```python
from build123d import *

# Parameters (mm, degrees)
SZKIC1_R                          = 10
DODANIE_WYCI_GNI_CIE1_DEPTH       = 357.5
SZKIC2_R                          = 8
DODANIE_WYCI_GNI_CIE2_DEPTH       = 32
SFAZOWANIE1_SIZE                  = 1.5
SFAZOWANIE2_SIZE2                 = 1.154700538
SFAZOWANIE2_SIZE                  = 2
SZKIC3_W                          = 28.491583868
SZKIC3_H                          = 26.39290166
SZKIC3_W_2                        = 17
SZKIC3_H_2                        = 17
WYTNIJ_WYCI_GNI_CIE1_DEPTH        = 5
SFAZOWANIE3_SIZE                  = 1
OTW_R_GWINTOWANY_M121_D           = 10.2
OTW_R_GWINTOWANY_M121_DEPTH       = 18
OTW_R_GWINTOWANY_M121_CSINK_D     = 13
OTW_R_GWINTOWANY_M121_CSINK_ANGLE = 90
OTW_R_GWINTOWANY_M121_TIP         = 3.064389157


with BuildPart() as part:
    # Szkic1 → Dodanie-wyciągnięcie1 (new body)
    with BuildSketch(Plane(origin=(0, 0, 0), x_dir=(0, 0, -1), z_dir=(1, 0, 0))):
        with Locations((-94.635912223, 0)):
            Circle(SZKIC1_R)
    extrude(amount=-DODANIE_WYCI_GNI_CIE1_DEPTH)

    # Szkic2 → Dodanie-wyciągnięcie2 (add)
    with BuildSketch(Plane.ZY.offset(357.5)):
        with Locations((94.635912223, 0)):
            Circle(SZKIC2_R)
    extrude(amount=DODANIE_WYCI_GNI_CIE2_DEPTH)

    # Sfazowanie1
    sfazowanie1_edges = [part.edges().sort_by_distance(p)[0] for p in [
        (-389.5, 0, 86.635912223),
    ]]
    chamfer(sfazowanie1_edges, length=SFAZOWANIE1_SIZE)

    # Sfazowanie2
    sfazowanie2_edges = [part.edges().sort_by_distance(p)[0] for p in [
        (-357.5, 0, 104.635912223),
    ]]
    sfazowanie2_side = [part.faces().sort_by_distance(p)[0] for p in [
        (-357.5, 0, 104.612818213),
    ]]
    chamfer(sfazowanie2_edges, length=SFAZOWANIE2_SIZE - 0.0001, length2=SFAZOWANIE2_SIZE2 - 0.0001, reference=sfazowanie2_side[0])  # a hair under: the kernel refuses the full size

    # Szkic3 → Wytnij-wyciągnięcie1 (cut)
    with BuildSketch(Plane.ZY.offset(357.5)):
        with Locations((94.635912223, 0)):
            Rectangle(SZKIC3_W, SZKIC3_H)
        with Locations((94.635912223, 0)):
            Rectangle(SZKIC3_W_2, SZKIC3_H_2, mode=Mode.SUBTRACT)
    extrude(amount=-WYTNIJ_WYCI_GNI_CIE1_DEPTH, mode=Mode.SUBTRACT)

    # Sfazowanie3
    sfazowanie3_edges = [part.edges().sort_by_distance(p)[0] for p in [
        (0, 0, 104.635912223),
    ]]
    chamfer(sfazowanie3_edges, length=SFAZOWANIE3_SIZE)

    # Otwór gwintowany M121
    with Locations(Plane(origin=(0, 0, 0), x_dir=(0, 0, -1), z_dir=(1, 0, 0))):
        with Locations((-94.635912223, 0)):
            CounterSinkHole(OTW_R_GWINTOWANY_M121_D / 2, OTW_R_GWINTOWANY_M121_CSINK_D / 2, depth=OTW_R_GWINTOWANY_M121_DEPTH, counter_sink_angle=OTW_R_GWINTOWANY_M121_CSINK_ANGLE)
            with Locations((0, 0, -(OTW_R_GWINTOWANY_M121_DEPTH + OTW_R_GWINTOWANY_M121_TIP / 2))):  # 118° drill point
                Cone(0, OTW_R_GWINTOWANY_M121_D / 2, OTW_R_GWINTOWANY_M121_TIP, mode=Mode.SUBTRACT)


solid = part.part
```
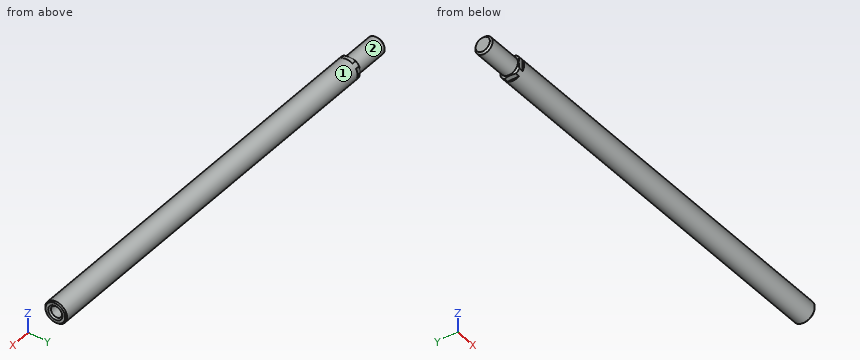
Read the model definition and answer for the solid it produces. Units are mm, in the model's axes. Face numbers are marked on the shaded views. A direction names the side the tool comes from. Round coordinates to 2 decimals unless told otherwise and drop trailing zeros. Loops run counter-clockwise (first coordinate to the right, second up) from the corner with the lowest first, then second, coordinate; pieces in that order, holes last. Notation, with made-up numbers: (62, -22) -> (115, -22) arc R27 ccw to (115, 3) -> close; hole circle Ø5 at (-22, 28.5). An arc over 180 degrees is marked (long way). One line per item, written item: value.
1) Flat-ended cylindrical pins translate along their axes: P1, Ø2.5, axis at x = -354.5, z = 94.5, coming from the +Y side; P2, Ø1.2, axis at y = 9.5, z = 96, coming from the -X side; P3, Ø1.4, axis at x = -354.5, y = 0, coming from the -Z side. Find the tip coordinate at first contact, or state that the pin passes through.
Answer list:
P1: stops at y = 8.5
P2: stops at x = -352.5
P3: stops at z = 86.14
2) For the marked faces 1 and 2, determine the directions among +Z, -Z, +X, -X, +Y, -Y from which every point of the face is accessible in a straight line to the end or side of a thin tool.
Answer list:
face 1: +X, -X
face 2: -X
3) A cutting plane is placed at A-A (x = -94). Determine the outline of the cut face in (y, z), and give its area (3 significant figures).
Answer list:
outline: circle Ø20 at (0, 94.64)
area: 314 mm²
4) Consider L1, parallel to Z at x = -9.75, y = 0; L2, parallel to Y at x = -126.5, z = 94; L3, parallel to X at y = -1, z = 88.25. Determine where each line is inside the solid, lowest interval first. Write a range as [from, to].
Answer list:
L1: z = [84.64, 89.54], [99.74, 104.64]
L2: y = [-9.98, 9.98]
L3: x = [-389.5, -0.04]
